```python
from build123d import *

# Parameters (mm, degrees)
SKETCH_1_R          = 35.2
SKETCH_1_R_2        = 24
EXTRUDE_1_DEPTH     = 13
SKETCH_2_R          = 2.505
CUT_EXTRUDE_1_DEPTH = 16
SKETCH_11_R         = 2.505
CUT_EXTRUDE_3_DEPTH = 16
SKETCH_12_R         = 2.505
CUT_EXTRUDE_4_DEPTH = 16


with BuildPart() as part:
    # 草圖1 → 伸長-薄件1 (new body)
    with BuildSketch(Plane(origin=(0, 0, 0), x_dir=(1, 0, 0), z_dir=(0, 1, 0))):
        Circle(SKETCH_1_R)
        Circle(SKETCH_1_R_2, mode=Mode.SUBTRACT)
    extrude(amount=EXTRUDE_1_DEPTH)

    # 草圖2 → 除料-伸長1 (cut)
    with BuildSketch(Plane(origin=(0, 0, 0), x_dir=(1, 0, 0), z_dir=(0, 1, 0))):
        with Locations((0, 26.330818465)):
            Circle(SKETCH_2_R)
    extrude(amount=CUT_EXTRUDE_1_DEPTH, mode=Mode.SUBTRACT)

    # 草圖11 → 除料-伸長3 (cut)
    with BuildSketch(Plane(origin=(0, 13, 0), x_dir=(1, 0, 0), z_dir=(0, 1, 0))):
        with Locations(Location((-16.103145177, -21.195220814, 0), (0, 0, 270))):
            Circle(SKETCH_11_R)
        with Locations(Location((15.916854823, -21.195220814, 0), (0, 0, 270))):
            Circle(SKETCH_11_R)
    extrude(amount=-CUT_EXTRUDE_3_DEPTH, mode=Mode.SUBTRACT)

    # 草圖12 → 除料-伸長4 (cut)
    with BuildSketch(Plane(origin=(0, 13, 0), x_dir=(1, 0, 0), z_dir=(0, 1, 0))):
        with Locations((-24.999999999, 7.794477134)):
            Circle(SKETCH_12_R)
        with Locations((25.000000001, 7.794477134)):
            Circle(SKETCH_12_R)
    extrude(amount=-CUT_EXTRUDE_4_DEPTH, mode=Mode.SUBTRACT)


solid = part.part
```
Design review of the part built by this model. Coordinates are the model's own, in mm. A direction names the side the tool comes from. Coordinates: 2 decimals unless noted, no trailing zeros. Order: outer loops, then holes, each group sorted by start corner. A loop starts at its lowest first (then second) coordinate and runs counter-clockwise, first axis right, second up. Notation, with made-up numbers: (3, -3.5) -> (11, -3.5) arc R10 cw to (11, 11.5) -> close; hole circle Ø11 at (27.5, -11.5). An arc over 180 degrees is marked (long way). One line per item, written item: value. Start each with the question number.
Q1. Take a section at B-B, the plane x = 0. State the section outline as (y, z) points.
Q2. Take a section at D-D, the plane x = -17. State the section outline as (y, z) points, then the cut area to 3 significant figures.
Q3. For probe 1 along X at (y, z) = (4.5, 0); probe 2 along Z at (x, y) = (-27, 9.5); probe 3 along X at (y, z) = (1.25, -5), list the stretches that pass through material, from the lowest coordinate up.
Q4. Take a section at C-C, the plane y = 9.5. State the section outline as (x, z) points (3 decimals).
Q5. Take a section at A-A, the plane z = 0. State the section outline as (x, y) points.
Q6. Insertion check: pin 1 Ø6 at (x, z) = (-11.5, -20.5) entering from +Y; pin 2 Ø4 at (x, z) = (-16.1, 21.2) entering from -Y; pin 3 Ø6 at (x, y) = (24.5, 2) entering from -Z. Each pin has a flat end and moves straight along its axis. Give the tip position at first contact, or say it passes through.
Q7. Tool access review of faces 1 (the flat face through (-8, 13, 23)), 2 (the cylindrical face through (14.264, 6.409, -19.301)): name each direction out of +Z, -Z, +X, -X, +Y, -Y from which nothing blocks a thin tool from reaching the whole face with its end or side.
Q8. Mouldability with a two-part tool opening along X and no side actions: class faces 3 (the cylindrical face through (33.575, 6.409, -10.573)), 4 (the flat face through (-8, 0, 23)), 5 (the cylindrical face through (-13.943, 6.409, -19.535)) as pulls with the +X half, pulls with the -X half, needs draft (parallel to the pull), parting line crosses it, or undercut.
Values follow:
1. outline: (0, -35.2) -> (13, -35.2) -> (13, -28.84) -> (0, -28.84) -> close; (0, 24) -> (13, 24) -> (13, 35.2) -> (0, 35.2) -> close
2. outline: (0, -30.82) -> (13, -30.82) -> (13, -16.94) -> (0, -16.94) -> close; (0, 16.94) -> (13, 16.94) -> (13, 18.86) -> (0, 18.86) -> close; (0, 23.53) -> (13, 23.53) -> (13, 30.82) -> (0, 30.82) -> close
2. area: 300 mm2
3. probe 1: x = -35.2 to -24, 24 to 35.2
3. probe 2: z = -22.58 to -9.3, -6.29 to 22.58
3. probe 3: x = -34.84 to -23.47, 23.47 to 34.84
4. outline: circle Ø70.4 at (0, 0); hole (-23.233, -6.019) arc R2.505 ccw (long way) to (-22.537, -8.251) arc R24 ccw to (-0.876, -23.984) arc R2.505 ccw (long way) to (0.876, -23.984) arc R24 ccw to (22.537, -8.251) arc R2.505 ccw (long way) to (23.233, -6.019) arc R24 ccw (long way) to start; hole circle Ø5.01 at (-16.103, 21.195); hole circle Ø5.01 at (15.917, 21.195)
5. outline: (-35.2, 0) -> (-24, 0) -> (-24, 13) -> (-35.2, 13) -> close; (24, 0) -> (35.2, 0) -> (35.2, 13) -> (24, 13) -> close
6. pin 1: stops at y = 13
6. pin 2: passes through
6. pin 3: stops at z = -27.87
7. face 1: +Z, -Z, +X, -X, +Y
7. face 2: +Y, -Y
8. face 3: parting line crosses it
8. face 4: needs draft
8. face 5: undercut
